Geometry check sheet. Reference: the model listing, model coordinates, mm. A direction names the side the tool comes from. Give positions to 0.01 mm unless a question says otherwise; leave off trailing zeros. Write each loop counter-clockwise with the first axis right and the second up, starting at its lowest first coordinate (ties: lowest second). Pieces come first, ordered by that corner, then holes. Notation, with made-up numbers: M 25,-19 L 64,-19 A13 ccw 64,-14 Z; hole C 60,13.25 d3. An arc over 180 degrees is marked long. One line per item, written item: value. Start each with the question number.
1. Cross-section at B-B on z = 0. Count the separate pieces of the cut face and the enclosed holes in it, then the cut area to 3 significant figures.
2. Tool access check on faces 4 (the face through (65, 1, 15)), 5 (the face through (25, 1, 12.5)), 6 (the face through (6, 1, 20)). Record the directions out of +Z, -Z, +X, -X, +Y, -Y that give a thin tool (end or side, any length) a straight path to the whole face; none if there is none.
3. Scan lines: line 1 (X direction, y = 1.7, z = 0); line 2 (Z direction, x = 26.5, y = 1); line 3 (Y direction, x = -1, z = 4). Record each from-to range of solid material in increasing order.
4. Release check for a two-part mould opening along Z. For faces 1 (the face through (-42.2, 5, 10.3)), 2 (the face through (10, 1, 11)), 3 (the face through (-41, 9, -2)) record: pulls with the +Z half, pulls with the -Z half, needs draft (parallel to the pull), parting line crosses it, or undercut.
5. Cross-section at C-C on y = 4.5. Record the cut outline in (x, z), then the cut area to 3 significant figures.
6. Gauge pin test, flat ends, axial feed: pin 1 (1.5 mm diameter, centred on y = 1, z = 11.5, fed in from -X); pin 2 (4 mm diameter, centred on y = 3.5, z = 11.5, fed in from -X); pin 3 (12 mm diameter, centred on x = 30, z = -14.5, fed in from +Y); pin 4 (6.5 mm diameter, centred on x = -52.5, z = 1.5, fed in from -Y). Record the tip position at first contact, or that the pin passes through.
7. Cross-section at A-A on x = 50. Record the cut outline in (y, z).
from build123d import *

# Parameters (mm, degrees)
CROQUIS1_R              = 11
CROQUIS1_R_2            = 2
CROQUIS1_W              = 30
CROQUIS1_H              = 3
SALIENTE_EXTRUIR1_DEPTH = 3
CROQUIS2_R              = 13
CROQUIS2_R_2            = 11
SALIENTE_EXTRUIR2_DEPTH = 4
CROQUIS3_R              = 13
CROQUIS3_R_2            = 9
SALIENTE_EXTRUIR3_DEPTH = 2
CHAFL_N1_SIZE           = 2
CHAFL_N2_SIZE           = 10


with BuildPart() as part:
    # Croquis1 → Saliente-Extruir1 (new body)
    with BuildSketch(Plane(origin=(0, 0, 0), x_dir=(1, 0, 0), z_dir=(0, 1, 0))):
        Polygon((65, 10), (70, 15), (70, -15), (65, -10), (65, -20), (-65, -20), (-65, 20), (65, 20), align=None)
        with Locations(Location((-50.129942902, 0, 0), (0, 0, 270))):
            Circle(CROQUIS1_R, mode=Mode.SUBTRACT)
        with Locations(Location((-28.595127909, 0, 0), (0, 0, 270))):
            Circle(CROQUIS1_R_2, mode=Mode.SUBTRACT)
        with Locations(Location((-13.595127909, 0, 0), (0, 0, 270))):
            Circle(CROQUIS1_R_2, mode=Mode.SUBTRACT)
        with Locations(Location((50, 0, 0), (0, 0, 270))):
            Circle(CROQUIS1_R_2, mode=Mode.SUBTRACT)
        with Locations((25, 11)):
            Rectangle(CROQUIS1_W, CROQUIS1_H, mode=Mode.SUBTRACT)
        with Locations((25, -11)):
            Rectangle(CROQUIS1_W, CROQUIS1_H, mode=Mode.SUBTRACT)
    extrude(amount=SALIENTE_EXTRUIR1_DEPTH)

    # Croquis2 → Saliente-Extruir2 (add)
    with BuildSketch(Plane(origin=(0, 3, 0), x_dir=(1, 0, 0), z_dir=(0, 1, 0))):
        with Locations(Location((-50.129942902, 0, 0), (0, 0, 90))):
            Circle(CROQUIS2_R)
        with Locations(Location((-50.129942902, 0, 0), (0, 0, 270))):
            Circle(CROQUIS2_R_2, mode=Mode.SUBTRACT)
    extrude(amount=SALIENTE_EXTRUIR2_DEPTH)

    # Croquis3 → Saliente-Extruir3 (add)
    with BuildSketch(Plane(origin=(0, 7, 0), x_dir=(1, 0, 0), z_dir=(0, 1, 0))):
        with Locations(Location((-50.129942902, 0, 0), (0, 0, 90))):
            Circle(CROQUIS3_R)
        with Locations(Location((-50.129942902, 0, 0), (0, 0, 270))):
            Circle(CROQUIS3_R_2, mode=Mode.SUBTRACT)
    extrude(amount=SALIENTE_EXTRUIR3_DEPTH)

    # Chaflán1
    chafl_n1_edges = [part.edges().sort_by_distance(p)[0] for p in [
        (-50.129942902, 9, 13),
    ]]
    chamfer(chafl_n1_edges, length=CHAFL_N1_SIZE)

    # Chaflán2
    chafl_n2_edges = [part.edges().sort_by_distance(p)[0] for p in [
        (-65, 1.5, 20),
        (-65, 1.5, -20),
    ]]
    chamfer(chafl_n2_edges, length=CHAFL_N2_SIZE)


solid = part.part
Report:
1. separate pieces: 5
1. enclosed holes: 0
1. area: 331 mm^2
2. face 4: +Z, +Y, -Y
2. face 5: +Y, -Y
2. face 6: +Z, +X, -X, +Y, -Y
3. line 1: x = -65 to -61.13, -39.13 to -30.6, -26.6 to -15.6, -11.6 to 48, 52 to 70
3. line 2: z = -20 to -12.5, -9.5 to 9.5, 12.5 to 20
3. line 3: y = 0 to 3
4. face 1: parting line crosses it
4. face 2: undercut
4. face 3: needs draft
5. outline: C -50.13,0 d26; hole C -50.13,0 d22
5. area: 151 mm^2
6. pin 1: stops at x = -64.25
6. pin 2: stops at x = -65
6. pin 3: stops at y = 3
6. pin 4: passes through
7. outline: M 0,-20 L 3,-20 L 3,-2 L 0,-2 Z; M 0,2 L 3,2 L 3,20 L 0,20 Z
